Check sheet for the modelled part. Datum: model origin and axes. Units: mm. A direction names the side the tool comes from. Give positions to 0.01 mm unless a question says otherwise; leave off trailing zeros. Write each loop counter-clockwise with the first axis right and the second up, starting at its lowest first coordinate (ties: lowest second). Pieces come first, ordered by that corner, then holes. Notation, with made-up numbers: (33.5, 63) -> (49.5, 63) arc R32 ccw to (49.5, 101) -> close; hole circle Ø1 at (62.5, 11.5). An arc over 180 degrees is marked (long way). Use a Markdown table: item, result. Add a question column.
1. Release check for a two-part mould opening along Y. For faces 1 (the flat face through (-38, -14, 1)), 2 (the flat face through (37, -7, 1)), 3 (the flat face through (17, 3, 1)), 4 (the flat face through (9, 2, 1)) record: released by +Y, released by -Y, zero draft, split by the parting line, or undercut.
2. Cross-section at A-A (y = -2). Enter the section's corners in (x, z), then the cut area to 3 significant figures.
3. Set-up check for faces 5 (the flat face through (-36, -3, 1)), 6 (the flat face through (-37, -21, 1)), 7 (the flat face through (32, 0, 1)), 8 (the flat face through (31, -28, 1)), 9 (the flat face through (39, -18, 1)): record each of +Z, -Z, +X, -X, +Y, -Y from which the full face is reachable in a straight line by a thin tool's end or side.
4. Scan lines: probe 1 along X at (y, z) = (0.5, 2.4); probe 2 along X at (y, z) = (-2, 0.65); probe 3 along Y at (x, z) = (27.5, 2.1). Record each from-to range of solid material in increasing order. Write a range as [from, to].
5. Gauge pin test, flat ends, axial feed: P1, Ø1.5, axis at x = 30.5, z = 2, coming from the +Y side; P2, Ø0.9, axis at y = -18.5, z = 1, coming from the -X side; P3, Ø1, axis at x = -5, y = -14.5, coming from the +Z side; P4, Ø1, axis at y = -9.5, z = 2, coming from the +X side. Record the tip position at first contact, or that the pin passes through.
from build123d import *

# Parameters (mm, degrees)
F1_DEPTH = 3


with BuildPart() as f1:
    # F0 (on Top) → F1 (new body)
    with BuildSketch(Plane.XY):
        with BuildLine():
            Line((-26, 0), (-36, 0))
            Line((-36, 0), (-36, -7))
            Line((-36, -7), (-39, -7))
            Line((-39, -7), (-39, -14))
            Line((-39, -14), (-36, -14))
            Line((-36, -14), (-36, -21))
            Line((-36, -21), (-39, -21))
            Line((-39, -21), (-39, -28))
            Line((-39, -28), (-26, -28))
            add(Edge.make_bspline(
                [(26, -28), (26, -12), (0, -12), (-26, -12), (-26, -28)],
                knots=[3.1415926536, 3.1415926536, 3.1415926536, 4.7123889804, 4.7123889804, 6.2831853072, 6.2831853072, 6.2831853072], degree=2, weights=[1, 0.7071067812, 1, 0.7071067812, 1]))
            Line((26, -28), (36, -28))
            Line((36, -28), (36, -21))
            Line((36, -21), (39, -21))
            Line((39, -21), (39, -14))
            Line((39, -14), (36, -14))
            Line((36, -14), (36, -7))
            Line((36, -7), (39, -7))
            Line((39, -7), (39, 0))
            Line((39, 0), (24, 0))
            Line((24, 0), (24, 3))
            Line((24, 3), (9, 3))
            Line((9, 3), (9, 0))
            Line((9, 0), (-11, 0))
            Line((-11, 0), (-11, 3))
            Line((-11, 3), (-26, 3))
            Line((-26, 3), (-26, 0))
        make_face()
    extrude(amount=F1_DEPTH)


solid = f1.part
Worked answers:
| question | item | result |
|---|---|---|
| 1 | face 1 | undercut |
| 1 | face 2 | undercut |
| 1 | face 3 | released by +Y |
| 1 | face 4 | zero draft |
| 2 | outline | (-36, 0) -> (39, 0) -> (39, 3) -> (-36, 3) -> close |
| 2 | area | 225 mm² |
| 3 | face 5 | +Z, -Z, -X, +Y |
| 3 | face 6 | +Z, -Z, -X |
| 3 | face 7 | +Z, -Z, +X, +Y |
| 3 | face 8 | +Z, -Z, +X, -X, -Y |
| 3 | face 9 | +Z, -Z, +X, +Y, -Y |
| 4 | probe 1 | x = [-26, -11], [9, 24] |
| 4 | probe 2 | x = [-36, 39] |
| 4 | probe 3 | y = [-28, 0] |
| 5 | P1 | stops at y = 0 |
| 5 | P2 | stops at x = -36 |
| 5 | P3 | passes through |
| 5 | P4 | stops at x = 36 |
